Build history of the part. All positions in model axes, mm. Give positions to 0.01 mm unless a question says otherwise; leave off trailing zeros. Loops run counter-clockwise (first coordinate to the right, second up) from the corner with the lowest first, then second, coordinate; pieces in that order, holes last. Notation, with made-up numbers: (-7, -5.75) -> (27, -5.75) arc R33 cw to (27, 29.25) -> close; hole circle Ø7 at (-30, 54.25). An arc over 180 degrees is marked (long way). Answer as a JSON object with one key per item and string values. Group by question number.
Q1. Band-saw the part on C-C, the plane y = 48.5. Write the cut outline in (x, z).
Q2. Wall check: probe 1 along X at (y, z) = (-32, 4); probe 2 along Y at (x, z) = (-34, 12); probe 3 along Y at (x, z) = (-47, 11.75). Give the ranges that are in metal, low to high. Write a range as from..to.
Q3. Band-saw the part on B-B, the plane x = -40.5. Write the cut outline in (y, z).
Q4. Band-saw the part on A-A, the plane z = 10. Write the cut outline in (x, y).
Q5. Drop flat-ended pins along their axis: pin 1 (1.5 mm diameter, centred on y = -37.5, z = 7, fed in from +X); pin 2 (1 mm diameter, centred on y = -29, z = 2.5, fed in from -X); pin 3 (4 mm diameter, centred on x = -37.5, z = 1.5, fed in from -Y). Give the stop position or say it passes through.
from build123d import *

# Parameters (mm, degrees)
F1_DEPTH = 12.7


with BuildPart() as f1:
    # F0 (on Top) → F1 (new body)
    with BuildSketch(Plane.XY):
        Polygon((-26.101787, -63.015288), (0, 0), (-63.015288, -26.101787), align=None)
        Polygon((26.101787, 63.015288), (-26.101787, 63.015288), (0, 0), align=None)
        Polygon((63.015288, 26.101787), (26.101787, 63.015288), (0, 0), align=None)
        Polygon((63.015288, 26.101787), (0, 0), (63.015288, -26.101787), align=None)
        Polygon((63.015288, -26.101787), (0, 0), (26.101787, -63.015288), align=None)
        Polygon((26.101787, -63.015288), (0, 0), (-26.101787, -63.015288), align=None)
        Polygon((0, 0), (-63.015288, 26.101787), (-63.015288, -26.101787), align=None)
        Polygon((0, 0), (-26.101787, 63.015288), (-63.015288, 26.101787), align=None)
    extrude(amount=F1_DEPTH)


solid = f1.part
Worked answers:
{
 "1": {"outline": "(-40.62, 0) -> (40.62, 0) -> (40.62, 12.7) -> (-40.62, 12.7) -> close"},
 "2": {"probe 1": "-57.12..57.12", "probe 2": "-55.12..55.12", "probe 3": "-42.12..42.12"},
 "3": {"outline": "(-48.62, 0) -> (48.62, 0) -> (48.62, 12.7) -> (-48.62, 12.7) -> close"},
 "4": {"outline": "(-63.02, -26.1) -> (-26.1, -63.02) -> (26.1, -63.02) -> (63.02, -26.1) -> (63.02, 26.1) -> (26.1, 63.02) -> (-26.1, 63.02) -> (-63.02, 26.1) -> close"},
 "5": {"pin 1": "x = 52.37", "pin 2": "x = -60.62", "pin 3": "y = -53.62"}
}
